Drawing for the job (mm, zero at the part's lowest x, y, z). Give positions to 0.01 mm unless a question says otherwise; leave off trailing zeros. Order: outer loops, then holes, each group sorted by start corner. A loop starts at its lowest first (then second) coordinate and runs counter-clockwise, first axis right, second up. Notation, with made-up numbers: (37, -5) -> (46, -5) arc R22 ccw to (46, 25) -> close; hole circle Ø6 at (-23.5, 40). An arc over 180 degrees is marked (long way). Use a Markdown table: item, result. Add a question column.
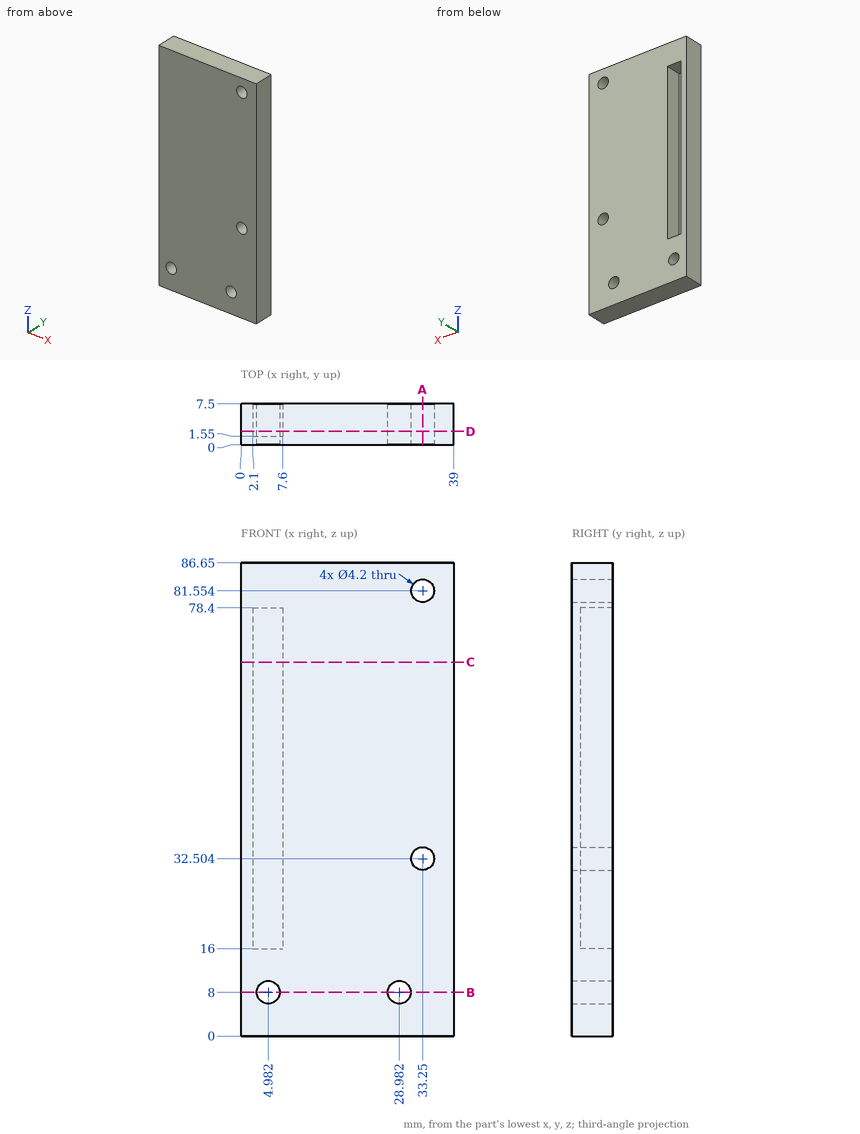
(1) Pin check, flat tip, straight feed: pin 1 Ø1.6 at (x, z) = (6, 44.5) entering from +Y. Stop position of the tip, or through.
(2) Band-saw the part on A-A on x = 33.25. Give the cut face in (y, z).
(3) Wall check: probe 1 along Z at (x, y) = (33.25, 2.5); probe 2 along X at (y, z) = (2.5, 8); probe 3 along X at (y, z) = (4.75, 35.5). Give the ranges that are in metal, low to high.
(4) Band-saw the part on B-B on z = 8. Give the cut face in (x, y), plus the area to 4 significant figures.
(5) Band-saw the part on C-C on z = 68.5. Give the cut face in (x, y), plus the area to 3 significant figures.
(6) Band-saw the part on D-D on y = 2.5. Give the cut face in (x, z), plus the area to 3 significant figures.
Response:
| question | item | result |
|---|---|---|
| 1 | pin 1 | stops at y = 1.55 |
| 2 | outline | (0, 0) -> (7.5, 0) -> (7.5, 30.4) -> (0, 30.4) -> close; (0, 34.6) -> (7.5, 34.6) -> (7.5, 79.45) -> (0, 79.45) -> close; (0, 83.65) -> (7.5, 83.65) -> (7.5, 86.65) -> (0, 86.65) -> close |
| 3 | probe 1 | z = 0 to 30.4, 34.6 to 79.45, 83.65 to 86.65 |
| 3 | probe 2 | x = 0 to 2.88, 7.08 to 26.88, 31.08 to 39 |
| 3 | probe 3 | x = 0 to 2.1, 7.6 to 39 |
| 4 | outline | (0, 0) -> (2.88, 0) -> (2.88, 7.5) -> (0, 7.5) -> close; (7.08, 0) -> (26.88, 0) -> (26.88, 7.5) -> (7.08, 7.5) -> close; (31.08, 0) -> (39, 0) -> (39, 7.5) -> (31.08, 7.5) -> close |
| 4 | area | 229.5 mm² |
| 5 | outline | (0, 0) -> (39, 0) -> (39, 7.5) -> (7.6, 7.5) -> (7.6, 1.55) -> (2.1, 1.55) -> (2.1, 7.5) -> (0, 7.5) -> close |
| 5 | area | 260 mm² |
| 6 | outline | (0, 0) -> (39, 0) -> (39, 86.65) -> (0, 86.65) -> close; hole (2.1, 16) -> (7.6, 16) -> (7.6, 78.4) -> (2.1, 78.4) -> close; hole circle Ø4.2 at (4.98, 8); hole circle Ø4.2 at (28.98, 8); hole circle Ø4.2 at (33.25, 32.5); hole circle Ø4.2 at (33.25, 81.55) |
| 6 | area | 2,980 mm² |
